Autodesk Inventor part; units mm, degrees
ref_plane "YZ Plane" through (0, 0, 0) normal (1, 0, 0) x (0, 1, 0)
ref_plane "XZ Plane" through (0, 0, 0) normal (0, 1, 0) x (-1, 0, 0)
ref_plane "XY Plane" through (0, 0, 0) normal (0, 0, 1) x (1, 0, 0)
sketch "Sketch1" plane through (0, 0, 0) normal (0, 1, 0) x (-1, 0, 0)
  line L0 (15, 20) -> (-15, 20)
  line L1 (-15, 20) -> (-15, -20)
  line L2 (-15, -20) -> (15, -20)
  line L3 (15, -20) -> (15, 20)
  line L4 (15, 20) -> (-15, -20) construction
  line L5 (-15, 20) -> (15, -20) construction
  point P0 (0, 0)
  dimension "d0" = 30
  dimension "d1" = 40
extrude "Extrusion1" add sketch "Sketch1" along normal blind 12
sketch "Sketch2" plane through (0, 12, 0) normal (0, 1, 0) x (1, 0, 0)
  line L0 (15, -20) -> (15, 20)
  line L1 (15, -12.5) -> (-2, -12.5)
  line L2 (-2, 8.5) -> (9, 8.5)
  line L3 (15, 8.5) -> (15, -12.5)
  line L4 (15, -10) -> (9, -10)
  line L5 (9, -10) -> (9, -12.5)
  line L6 (9, -12.5) -> (15, -12.5)
  line L7 (15, -12.5) -> (15, -10)
  line L8 (-2, -12.5) -> (-7, -12.5)
  line L9 (-7, -12.5) -> (-7, -8.5)
  line L10 (-7, -8.5) -> (-2, -8.5)
  line L11 (-2, -8.5) -> (-2, -12.5)
  line L12 (-2, -4) -> (-7, -4)
  line L13 (-7, -4) -> (-7, 0)
  line L14 (-7, 0) -> (-2, 0)
  line L15 (-2, 8.5) -> (-7, 8.5)
  line L16 (-7, 8.5) -> (-7, 4.5)
  line L17 (-7, 4.5) -> (-2, 4.5)
  line L18 (-2, 4.5) -> (-2, 8.5)
  line L19 (15, 8.5) -> (9, 8.5)
  line L20 (9, 8.5) -> (9, 12.5)
  line L21 (9, 12.5) -> (15, 12.5)
  line L22 (15, 12.5) -> (15, 8.5)
  line L23 (-2, -8.5) -> (-2, -4)
  line L24 (-2, 0) -> (-2, 4.5)
  line L25 (-15, -20) -> (15, -20)
  line L26 (15, 20) -> (-15, 20)
  point P0 (0, 0)
  point P1 (15, -10)
  dimension "d4" = 21
  dimension "d5" = 17
  dimension "d7" = 2.5
  dimension "d8" = 5
  dimension "d9" = 4
  dimension "d10" = 4
  dimension "d11" = 4
  dimension "d12" = 4.5
  dimension "d13" = 4.5
  dimension "d14" = 4
  dimension "d15" = 7.5
  dimension "d22" = 25
  dimension "d23" = 7.5
extrude "Extrusion2" cut sketch "Sketch2" against normal blind 6.5 contours L4 L5 L1 L11 L23 L12 L13 L14 L24 L18 L2 L19 L0 | L19 L20 L21 L0 | L8 L9 L10 L11 | L18 L17 L16 L15
move faces "Move1" translate (-4, 0, 0) faces at (-7, 9.8333, 9.8333) (-7, 9.8333, 1.3333) (-7, 9.8333, -7.1667)
fillet "Fillet1" radius 5 4 edges at (-15, 6, -20) (-15, 6, 20) (15, 6, -20) (15, 6, 20)
equation "\"d10\" = d9"
equation "\"d11\" = d9"
equation "\"d13\" = d12"
equation "\"d15\" = d23"
properties part number "wooden_limitswitch"
CAD build for the part. Positions are in the model's coordinates, mm. A direction names the side the tool comes from. Coordinates: 2 decimals unless noted, no trailing zeros. Loops run counter-clockwise (first coordinate to the right, second up) from the corner with the lowest first, then second, coordinate; pieces in that order, holes last. Notation, with made-up numbers: (80, 67.25) - (134, 67.25) arc R10 cw to (134, 71.25) - close; hole circle Ø10 at (47.25, 80). An arc over 180 degrees is marked (long way). Write item = value, one per line. Start each with the question number.
Q1. Flat gauge pins, fed straight in: pin 1 Ø1 at (x, y) = (-10.5, 4) entering from -Z; pin 2 Ø1.3 at (y, z) = (7.5, -1) entering from +X; pin 3 Ø1.2 at (y, z) = (8.5, 2.5) entering from +X; pin 4 Ø4.5 at (y, z) = (9.5, -10) entering from +X. Where does each tip first touch, or does it go through?
Q2. Which spindle directions (+Z, -Z, +X, -X, +Y, -Y) get a long thin tool onto all of the face, cutting with end or side? Do faces 5 (the flat face through (0, 6, 20)), 6 (the flat face through (9, 9, -10)), 7 (the flat face through (-1, 9, 12.5)). Say none if no direction does.
Q3. Cut at C-C, the plane y = 10.5. List the corners of the cut face in (x, z), then the cut area to 3 significant figures.
Q4. Cut at D-D, the plane x = 7.25. List the corners of the cut face in (y, z).
Q5. Cut at B-B, the plane z = 2.5. List the corners of the cut face in (x, y), then the cut area to 3 significant figures.
Q6. Cut at A-A, the plane x = -8.75. List the corners of the cut face in (y, z), then the cut area to 3 significant figures.
Q7. Pull direction Z, two halves, no side cores. Call faces 1 (the cylindrical face through (-14, 6, -18)), 2 (the flat face through (-11, 9, 11)), 3 (the flat face through (-15, 6, 0)), 4 (the flat face through (-11, 9, 2)): pulls with the +Z half, pulls with the -Z half, needs draft (parallel to the pull), parting line crosses it, or undercut.
Q8. Drill centre lines: L1, parallel to Z at x = -9, y = 7; L2, parallel to X at y = 8.25, z = 12; L3, parallel to Z at x = 8.25, y = 8.25. Where is each one in solid material? Low to high.
Computed:
q1.pin_1 = -20
q1.pin_2 = -2
q1.pin_3 = -11
q1.pin_4 = 9
q2.face_5 = +Z, +X, -X, +Y, -Y
q2.face_6 = +X, +Y
q2.face_7 = +Y
q3.outline = (-15, -15) arc R5 ccw to (-10, -20) - (10, -20) arc R5 ccw to (15, -15) - (15, -12.5) - (9, -12.5) - (9, -8.5) - (-11, -8.5) - (-11, -4.5) - (-2, -4.5) - (-2, 0) - (-11, 0) - (-11, 4) - (-2, 4) - (-2, 8.5) - (-11, 8.5) - (-11, 12.5) - (9, 12.5) - (9, 10) - (15, 10) - (15, 15) arc R5 ccw to (10, 20) - (-10, 20) arc R5 ccw to (-15, 15) - close
q3.area = 705 mm²
q4.outline = (0, -20) - (12, -20) - (12, -8.5) - (5.5, -8.5) - (5.5, 12.5) - (12, 12.5) - (12, 20) - (0, 20) - close
q5.outline = (-15, 0) - (15, 0) - (15, 5.5) - (-11, 5.5) - (-11, 12) - (-15, 12) - close
q5.area = 191 mm²
q6.outline = (0, -20) - (12, -20) - (12, -8.5) - (5.5, -8.5) - (5.5, -4.5) - (12, -4.5) - (12, 0) - (5.5, 0) - (5.5, 4) - (12, 4) - (12, 8.5) - (5.5, 8.5) - (5.5, 12.5) - (12, 12.5) - (12, 20) - (0, 20) - close
q6.area = 402 mm²
q7.face_1 = pulls with the -Z half
q7.face_2 = undercut
q7.face_3 = needs draft
q7.face_4 = undercut
q8.L1 = -20 to -8.5, -4.5 to 0, 4 to 8.5, 12.5 to 20
q8.L2 = -15 to -11, 9 to 15
q8.L3 = -20 to -8.5, 12.5 to 20
